Could you check a few things on this model? Use its own coordinates, in mm. A direction names the side the tool comes from. Give positions to 0.01 mm unless a question says otherwise; leave off trailing zeros. Order: outer loops, then holes, each group sorted by start corner. A loop starts at its lowest first (then second) coordinate and runs counter-clockwise, first axis right, second up. Notation, with made-up numbers: (-12.75, -33) -> (-4.75, -33) arc R19 cw to (-4.75, -6) -> close; hole circle Ø11 at (-29, 50.25). An arc over 180 degrees is marked (long way). Answer as CSV lines item,"result". Start each with the question number.
(1) On a 3-axis mill with a long thin cutter (end or side, diameter ignored), from which of +Z, -Z, +X, -X, +Y, -Y can I reach the whole of each face in a straight line? I mean faces 1 (the face through (10, -10, 5)), 2 (the face through (0, 3, 505)). Say none if no direction works.
(2) I want a section at A-A (z = 176.5). Please give me the cut outline in (x, y).
(3) I want a section at B-B (y = 29.5). Please give me the cut outline in (x, z), plus the area to 3 significant figures.
(4) Will these pins go through, and if not, where does the flat tip stop? pin 1 Ø12 at (y, z) = (-12.5, 260.5) entering from +X; pin 2 Ø12 at (x, z) = (4.5, 425) entering from -Y; pin 3 Ø10 at (x, y) = (-17.5, -31.5) entering from +Z.
(5) I need wall thicknesses on L1, parallel to Y at x = 0, z = 501; L2, parallel to Z at x = -44, y = -14. Which ranges of each line are inside material? Lowest first, please.
(6) I want a section at C-C (x = -32.5). Please give me the cut outline in (y, z), plus the area to 3 significant figures.
Autodesk Fusion 360 part; units mm, degrees
sketch "Sketch1" plane through (0, 0, 0) normal (0, 0, 1) x (1, 0, 0)
  circle A0 centre (0, 0) radius 50
  dimension "d1" = 100
extrude "Extrude1" add sketch "Sketch1" along normal blind 5
sketch "Sketch2" plane through (0, 0, 5) normal (0, 0, 1) x (-1, 0, 0)
  circle A0 centre (0, 0) radius 50
  circle A1 centre (0, 0) radius 12.5
  dimension "d4" = 25
extrude "Extrude2" add sketch "Sketch2" along normal blind 500 contours A1
sketch "Sketch3" plane through (0, 0, 505) normal (0, 0, 1) x (-1, 0, 0)
  circle A0 centre (0, 0) radius 12.5
  circle A1 centre (0, 0) radius 2.5
  dimension "d7" = 5
extrude "Extrude3" cut sketch "Sketch3" against normal blind 10 contours A1
Final values:
1,face 1,"+Z"
1,face 2,"+Z, +X, -X, +Y, -Y"
2,outline,"circle Ø25 at (0, 0)"
3,outline,"(-40.37, 0) -> (40.37, 0) -> (40.37, 5) -> (-40.37, 5) -> close"
3,area,"404 mm²"
4,pin 1,"x = 10.68"
4,pin 2,"y = -12.5"
4,pin 3,"z = 5"
5,L1,"-12.5 to -2.5, 2.5 to 12.5"
5,L2,"0 to 5"
6,outline,"(-38, 0) -> (38, 0) -> (38, 5) -> (-38, 5) -> close"
6,area,"380 mm²"
